Part model, mm, in its own coordinate system. A direction names the side the tool comes from. Give positions to 0.01 mm unless a question says otherwise; leave off trailing zeros. Order: outer loops, then holes, each group sorted by start corner. A loop starts at its lowest first (then second) coordinate and runs counter-clockwise, first axis right, second up. Notation, with made-up numbers: M 26,-27 L 51,-27 A26 ccw 51,10 Z; hole C 64.5,-37 d6. An arc over 180 degrees is marked long. Write each question's results on one line, items separated by ' | '. Start each with the question number.
from build123d import *

# Parameters (mm, degrees)
F0_R            = 42.5
F0_R_2          = 25
F1_DEPTH        = 15
F2_DEPTH        = 50
F3_SIZE         = 1
F4_R            = 12.5
F5_DEPTH        = 50.001
F6_SIZE         = 2
F7_R            = 3.25
F8_DEPTH        = 50.001
F8_COPIES_COUNT = 3
F7_R_2          = 6
F9_DEPTH        = 8
F9_COPIES_COUNT = 3
F10_SIZE        = 0.5


# Not quite as in the source:
# - a pattern or mirror of a feature is missing from the dataset's text; its kind, count and spacing are read off the source's solid


with BuildPart() as f1:
    # F0 (on Front) → F1 (new body)
    with BuildSketch(Plane.XZ):
        Circle(F0_R)
        Circle(F0_R_2, mode=Mode.SUBTRACT)
        Circle(F0_R_2)
    extrude(amount=F1_DEPTH)

    # F0 (on Front) → F2 (join)
    with BuildSketch(Plane.XZ):
        Circle(F0_R_2)
    extrude(amount=F2_DEPTH)

    # F3
    f3_edges = [f1.edges().sort_by_distance(p)[0] for p in [
        (-42.5, 0, 0),
        (-42.5, -15, 0),
        (-25, -50, 0),
    ]]
    chamfer(f3_edges, length=F3_SIZE)

    # F4 (on face) → F5 (cut, through all)
    with BuildSketch(Plane.XZ.offset(50)):
        Circle(F4_R)
    extrude(amount=-F5_DEPTH, mode=Mode.SUBTRACT)

    # F6
    f6_edges = [f1.edges().sort_by_distance(p)[0] for p in [
        (-12.5, -50, 0),
        (-12.5, 0, 0),
    ]]
    chamfer(f6_edges, length=F6_SIZE)

    # F7 (on face) → F8 (cut, through all)
    with BuildSketch(Plane(origin=(0, 0, 0), x_dir=(-1, 0, 0), z_dir=(0, 1, 0))):
        with Locations((32.5, 0)):
            Circle(F7_R)
    f8 = extrude(amount=-F8_DEPTH, mode=Mode.SUBTRACT)

    # F8_copies: F8 ×3 about axis
    f8_copies_axis = Axis((0, 0, 0), (0, 1, 0))
    for i in range(1, F8_COPIES_COUNT):
        add(f8.rotate(f8_copies_axis, i * 360 / F8_COPIES_COUNT), mode=Mode.SUBTRACT)

    # F7 (on face) → F9 (cut)
    with BuildSketch(Plane(origin=(0, 0, 0), x_dir=(-1, 0, 0), z_dir=(0, 1, 0))):
        with Locations((32.5, 0)):
            Circle(F7_R_2)
        with Locations((32.5, 0)):
            Circle(F7_R, mode=Mode.SUBTRACT)
    f9 = extrude(amount=-F9_DEPTH, mode=Mode.SUBTRACT)

    # F9_copies: F9 ×3 about axis
    f9_copies_axis = Axis((0, 0, 0), (0, 1, 0))
    for i in range(1, F9_COPIES_COUNT):
        add(f9.rotate(f9_copies_axis, i * 360 / F9_COPIES_COUNT), mode=Mode.SUBTRACT)

    # F10
    f10_edges = [f1.edges().sort_by_distance(p)[0] for p in [
        (-26.5, 0, 0),
        (-29.25, -15, 0),
        (13.25, 0, -22.949673),
        (13.25, 0, 22.949673),
        (14.625, -15, -25.331243),
        (14.625, -15, 25.331243),
    ]]
    chamfer(f10_edges, length=F10_SIZE)


solid = f1.part
(1) Drop flat-ended pins along their axis: P1, Ø6, axis at y = -17, z = -14, coming from the -X side; P2, Ø3.5, axis at x = 15.5, z = -25, coming from the +Y side; P3, Ø5, axis at x = 20.5, y = -29, coming from the +Z side; P4, Ø14, axis at x = -32.5, z = 0, coming from the +Y side. Give the stop position or say it passes through.
(2) Tool access for faces 5 (the cylindrical face through (-27.74, -4.2, -3.65)), 6 (the cylindrical face through (23.846, -31.762, 7.509)), 7 (the cylindrical face through (14.503, -11.204, 30.886)): list every direction of +Z, -Z, +X, -X, +Y, -Y with a clear straight run to the whole face (end or side of a thin tool).
(3) Saw through at B-B on y = -12.5. Give the cut face in (x, z) (3 decimals), plus the area to 3 significant figures.
(4) Saw through at A-A on x = 0. Give the cut face in (y, z).
(5) Probe L1, parallel to Z at x = 16.25, y = -11.25; L2, parallel to Y at x = -9.5, z = -26.5; L3, parallel to Z at x = -7, y = -27. List the from-to ranges inside material, lowest first.
(6) Pull direction Z, two halves, no side cores. Call faces 1 (the flat face through (15, -8, 32)), 2 (the cylindrical face through (-33.727, -7.409, -25.861)), 3 (the flat face through (18, -15, -18)), 4 (the cylindrical face through (16.673, -11.204, -24.923)): +Z half, -Z half, draft (parallel to the pull), parting line (faces both ways), or undercut.
(7) Saw through at C-C on x = 16.25. Give the number of separate pieces and of enclosed holes in the cut face, plus the area to 3 significant figures.
Taken from the geometry:
1) P1: stops at x = -40.29 | P2: stops at y = -8 | P3: stops at z = 17.35 | P4: stops at y = 0
2) face 5: +Y | face 6: -Y | face 7: +Y, -Y
3) outline: C 0,0 d85; hole C -32.5,0 d6.5; hole C 0,0 d25; hole C 16.25,-28.146 d6.5; hole C 16.25,28.146 d6.5 | area: 5,080 mm²
4) outline: M -50,-24 L -49,-25 L -15,-25 L -15,-41.5 L -14,-42.5 L -1,-42.5 L 0,-41.5 L 0,-14.5 L -2,-12.5 L -48,-12.5 L -50,-14.5 Z; M -50,14.5 L -48,12.5 L -2,12.5 L 0,14.5 L 0,41.5 L -1,42.5 L -14,42.5 L -15,41.5 L -15,25 L -49,25 L -50,24 Z
5) L1: z = -39.27 to -31.4, -24.9 to 24.9, 31.4 to 39.27 | L2: y = -15 to 0 | L3: z = -24 to -10.36, 10.36 to 24
6) face 1: undercut | face 2: parting line | face 3: draft | face 4: undercut
7) separate pieces: 3 | enclosed holes: 0 | area: 2,220 mm²
